Geometry check sheet. Reference: drawing and pictorial views, mm from the part's lowest x, y, z. Round coordinates to 2 decimals unless told otherwise and drop trailing zeros. Order: outer loops, then holes, each group sorted by start corner. A loop starts at its lowest first (then second) coordinate and runs counter-clockwise, first axis right, second up.
(1) Depth check by flat-ended pin: pin 1 (3 mm diameter, centred on y = 59.5, z = 2.5, fed in from -X) (1 decimal); pin 2 (1.5 mm diameter, centred on y = 85, z = 2.5, fed in from +X); pin 3 (1.5 mm diameter, centred on y = 38.5, z = 4, fed in from +X). Enter the tip coordinate at first touch or a pass-through.
(2) Sectioned sample at A-A, the plane x = 40.5. Enter the section's corners in (y, z) (1 decimal).
(3) Thickness scan on probe 1 along Z at (x, y) = (7.5, 75.5); probe 2 along X at (y, z) = (17, 3.9); probe 3 along X at (y, z) = (79, 1.45) (1 decimal). Record the ranges inside material, lowest first.
(4) Mould release check, pull along Z, two halves, no side actions. Record for the marked faces 1 and 2: released by +Z, released by -Z, zero draft, split by the parting line, or undercut.
(5) Sectioned sample at B-B, the plane y = 83.5. Enter the section's corners in (x, z) (1 decimal).
(6) Sectioned sample at C-C, the plane z = 1. Count the separate pieces of the cut face and the enclosed holes in it, and give its area (3 significant figures).
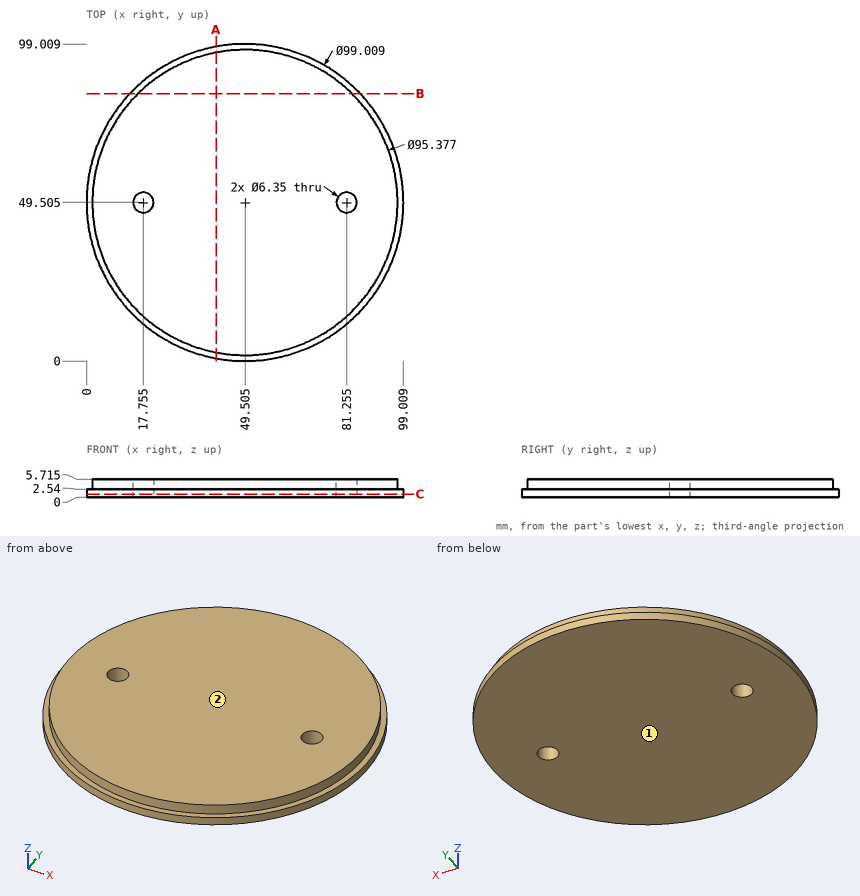
Derived:
1. pin 1: stops at x = 0.7
1. pin 2: stops at x = 84.77
1. pin 3: stops at x = 96.08
2. outline: (0.8, 0) - (98.2, 0) - (98.2, 2.5) - (96.3, 2.5) - (96.3, 5.7) - (2.7, 5.7) - (2.7, 2.5) - (0.8, 2.5) - close
3. probe 1: z = 0 to 2.54
3. probe 2: x = 14.61 to 84.4
3. probe 3: x = 9.7 to 89.3
4. face 1: released by -Z
4. face 2: released by +Z
5. outline: (13.5, 0) - (85.5, 0) - (85.5, 2.5) - (82.9, 2.5) - (82.9, 5.7) - (16.1, 5.7) - (16.1, 2.5) - (13.5, 2.5) - close
6. separate pieces: 1
6. enclosed holes: 2
6. area: 7,640 mm2
